Source: CAD feature listing. Evaluate the final solid. Frame: model axes, mm. Face numbers are marked on the shaded views. A direction names the side the tool comes from. Coordinates: 2 decimals unless noted, no trailing zeros. Write each loop counter-clockwise with the first axis right and the second up, starting at its lowest first coordinate (ties: lowest second). Pieces come first, ordered by that corner, then holes. Notation, with made-up numbers: (47, 67.5) - (58, 67.5) arc R17 ccw to (58, 86.5) - close; hole circle Ø4 at (-9.75, -15). An arc over 180 degrees is marked (long way). One line per item, written item: value.
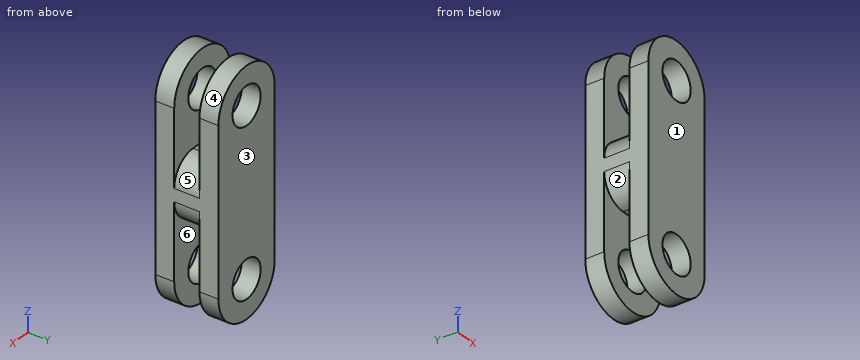
Autodesk Inventor part; units mm, degrees
ref_plane "YZ Plane" through (0, 0, 0) normal (1, 0, 0) x (0, 1, 0)
ref_plane "XZ Plane" through (0, 0, 0) normal (0, 1, 0) x (-1, 0, 0)
ref_plane "XY Plane" through (0, 0, 0) normal (0, 0, 1) x (1, 0, 0)
sketch "Sketch1" plane through (0, 0, 0) normal (0, 1, 0) x (-1, 0, 0)
  line L0 (-3, 10) -> (3, 10)
  line L1 (3, 10) -> (3, -10)
  line L2 (3, -10) -> (-3, -10)
  line L3 (-3, -10) -> (-3, 10)
  line L4 (-3, 10) -> (3, -10) construction
  line L5 (3, 10) -> (-3, -10) construction
  line L6 (0, -10) -> (0, -6.5) construction
  line L7 (0, 10) -> (0, 6.5) construction
  circle A0 centre (0, 6.5) radius 1.5
  circle A1 centre (0, -6.5) radius 1.5
  point P0 (0, 0)
  dimension "d0" = 6
  dimension "d1" = 20
  dimension "d2" = 3.5
  dimension "d3" = 3.5
  dimension "d4" = 3
  dimension "d5" = 3
extrude "Extrusion1" add sketch "Sketch1" along normal blind 1.5
fillet "Fillet1" radius 2 4 edges at (3, 0.75, 10) (-3, 0.75, 10) (3, 0.75, -10) (-3, 0.75, -10)
sketch "Sketch2" plane through (0, 1.5, 0) normal (0, 1, 0) x (1, 0, 0)
  circle A0 centre (0, -6.5) radius 1.5
  circle A1 centre (0, -6.5) radius 1.5
  circle A2 centre (0, -6.5) radius 3
  line L0 (-3, -6.5) -> (3, -6.5)
  line L1 (3, -6.5) -> (3, -10)
  line L2 (3, -10) -> (-3, -10)
  line L3 (-3, -10) -> (-3, -6.5)
  point P0 (0, 0)
  point P1 (3, -6.5)
  dimension "d9" = 6
  dimension "d10" = 3
  dimension "d11" = 3.5
extrude "Extrusion2" cut sketch "Sketch2" against normal through all contours L1 L2 L3 A2
mirror "Mirror1" about plane through (0, 0, 0) normal (0, 0, 1) of "Extrusion2"
sketch "Sketch3" plane through (0, 1.5, 0) normal (0, 1, 0) x (1, 0, 0)
  line L0 (-3, 6.5) -> (-3, -6.5)
  line L1 (3, -2.5) -> (-3, -2.5)
  line L2 (-3, -2.5) -> (-3, 2.5)
  line L3 (-3, 2.5) -> (3, 2.5)
  line L4 (3, 2.5) -> (3, -2.5)
  line L5 (3, -2.5) -> (-3, 2.5) construction
  line L6 (-3, -2.5) -> (3, 2.5) construction
  point P0 (0, 0)
  dimension "d14" = 5
extrude "Extrusion3" add sketch "Sketch3" along normal blind 2
ref_plane "Work Plane1" through (0, 2.5, 0) normal (0, -1, 0) x (1, 0, 0)
mirror "Mirror2" about plane through (0, 2.5, 0) normal (0, -1, 0) of "Extrusion1", "Fillet1", "Extrusion2", "Mirror1"
fillet "Fillet2" radius 2 4 edges at (3, 2.5, 2.5) (3, 2.5, -2.5) (-3, 2.5, 2.5) (-3, 2.5, -2.5)
properties part number "DAWN_chain_round"
1) Material intervals for line 1 (Z direction, x = 0, y = 4.65); line 2 (Y direction, x = 1.6, z = -6.75); line 3 (Z direction, x = 0.45, y = 3.85), sorted ascending.
Values found:
line 1: -9.5 to -8, -5 to 5, 8 to 9.5
line 2: 0 to 1.5, 3.5 to 5
line 3: -9.47 to -7.93, -5.07 to 5.07, 7.93 to 9.47
2) Draft query along Y for the marked faces 3, 4, 5 and 6. Return one class per face: released by +Y, released by -Y, zero draft, split by the parting line, or undercut.
Values found:
face 3: released by +Y
face 4: zero draft
face 5: undercut
face 6: undercut
3) Reachability of the marked faces 1 and 2 from +Z, -Z, +X, -X, +Y, -Y: full face, straight path, thin tool, end or side. Return the list, or none.
Values found:
face 1: +Z, -Z, +X, -X, -Y
face 2: -Z, -X
4) Section query B-B on z = -4. Output: boundary loops of the cut face in (x, y).
Values found:
outline: (-3, 0) - (3, 0) - (3, 1.5) - (-3, 1.5) - close; (-3, 3.5) - (3, 3.5) - (3, 5) - (-3, 5) - close
5) Section query C-C on y = 2. Output: boundary loops of the cut face in (x, z), then the cut area to 3 significant figures.
Values found:
outline: (-3, -0.5) arc R2 ccw to (-1, -2.5) - (1, -2.5) arc R2 ccw to (3, -0.5) - (3, 0.5) arc R2 ccw to (1, 2.5) - (-1, 2.5) arc R2 ccw to (-3, 0.5) - close
area: 26.6 mm2
6) Section query A-A on x = 0. Output: boundary loops of the cut face in (y, z).
Values found:
outline: (0, -9.5) - (1.5, -9.5) - (1.5, -8) - (0, -8) - close; (0, -5) - (1.5, -5) - (1.5, -2.5) - (3.5, -2.5) - (3.5, -5) - (5, -5) - (5, 5) - (3.5, 5) - (3.5, 2.5) - (1.5, 2.5) - (1.5, 5) - (0, 5) - close; (0, 8) - (1.5, 8) - (1.5, 9.5) - (0, 9.5) - close; (3.5, -9.5) - (5, -9.5) - (5, -8) - (3.5, -8) - close; (3.5, 8) - (5, 8) - (5, 9.5) - (3.5, 9.5) - close
7) Section query D-D on z = -6.25. Output: boundary loops of the cut face in (x, y), then the cut area to 3 significant figures.
Values found:
outline: (-3, 0) - (-1.48, 0) - (-1.48, 1.5) - (-3, 1.5) - close; (-3, 3.5) - (-1.48, 3.5) - (-1.48, 5) - (-3, 5) - close; (1.48, 0) - (3, 0) - (3, 1.5) - (1.48, 1.5) - close; (1.48, 3.5) - (3, 3.5) - (3, 5) - (1.48, 5) - close
area: 9.13 mm2
